```python
from build123d import *

# Parameters (mm, degrees)
SKETCH1_W           = 30
SKETCH1_H           = 15
BOSS_EXTRUDE1_DEPTH = 10
BOSS_EXTRUDE2_DEPTH = 15
FILLET1_R           = 3
SKETCH3_R           = 1.25
CUT_EXTRUDE1_DEPTH  = 11
SKETCH4_R           = 1.25
CUT_EXTRUDE2_DEPTH  = 16.0000001


with BuildPart() as part:
    # Sketch1 → Boss-Extrude1 (new body)
    with BuildSketch(Plane(origin=(0, 0, 0), x_dir=(1, 0, 0), z_dir=(0, 1, 0))):
        Rectangle(SKETCH1_W, SKETCH1_H)
    extrude(amount=BOSS_EXTRUDE1_DEPTH)

    # Sketch2 → Boss-Extrude2 (add)
    with BuildSketch(Plane.XZ):
        Polygon((-13, -5.5), (-4, -5.5), (-4, -1.5), (4, -1.5), (4, -5.5), (13, -5.5), (13, 5.5), (4, 5.5), (4, 1.5), (-4, 1.5), (-4, 5.5), (-13, 5.5), align=None)
    extrude(amount=BOSS_EXTRUDE2_DEPTH)

    # Fillet1
    fillet1_edges = [part.edges().sort_by_distance(p)[0] for p in [
        (-15, 10, 0),
        (0, 10, 7.5),
        (13, -7.5, 5.5),
        (-13, -7.5, 5.5),
        (-13, -7.5, -5.5),
        (13, -7.5, -5.5),
        (15, 10, 0),
        (15, 5, 7.5),
        (-15, 5, 7.5),
        (-15, 5, -7.5),
        (15, 5, -7.5),
        (0, 10, -7.5),
    ]]
    fillet(fillet1_edges, radius=FILLET1_R)

    # Sketch3 → Cut-Extrude1 (cut, through all)
    with BuildSketch(Plane.XZ):
        with Locations((0, 3.5)):
            Circle(SKETCH3_R)
        with Locations((0, -3.5)):
            Circle(SKETCH3_R)
    extrude(amount=-CUT_EXTRUDE1_DEPTH, mode=Mode.SUBTRACT)

    # Sketch4 → Cut-Extrude2 (cut, through all)
    with BuildSketch(Plane.XY.offset(7.5)):
        with Locations((0, 5)):
            Circle(SKETCH4_R)
    extrude(amount=-CUT_EXTRUDE2_DEPTH, mode=Mode.SUBTRACT)


solid = part.part
```
The model under review builds one solid part; all positions refer to its coordinate system, in mm. A direction names the side the tool comes from. Round coordinates to 2 decimals unless told otherwise and drop trailing zeros. Loops run counter-clockwise (first coordinate to the right, second up) from the corner with the lowest first, then second, coordinate; pieces in that order, holes last. Notation, with made-up numbers: (59, 12) - (112, 12) arc R24 ccw to (112, 27) - close; hole circle Ø2 at (68.5, -16.5). An arc over 180 degrees is marked (long way). Write each question's results on one line, items separated by ' | '. Start each with the question number.
Q1. Insertion check: P1, Ø4, axis at x = 1.5, y = -4.5, coming from the -Z side; P2, Ø4, axis at x = -11, y = -5.5, coming from the +Z side; P3, Ø4.5, axis at y = -7.5, z = 2.5, coming from the +X side. Each pin has a flat end and moves straight along its axis. Give the tip position at first contact, or say it passes through.
Q2. Take a section at D-D on y = 1.25. Give the boundary of the cut face in (x, z), plus the area to 3 significant figures.
Q3. Draft analysis for pull direction X (two halves, no side actions). For faces 1 (the cylindrical face through (-1.25, 1.91, -3.45)), 2 (the cylindrical face through (1.155, 4.521, 5.972)), 3 (the cylindrical face through (0.17, 9.1, -6.64)), 4 (the flat face through (-15, 3, 0)), state which applies: pulls with the +X half, pulls with the -X half, needs draft (parallel to the pull), parting line crosses it, or undercut.
Q4. Wall thickness on line 1 along Z through (x, y) = (0, 6.8); line 2 along X through (y, z) = (1.05, 3.5); line 3 along X through (y, z) = (-7.25, 2): over which ranges is each line inside the solid? List them lowest first. Write a range as [from, to].
Q5. Take a section at B-B on y = -5.75. Give the boundary of the cut face in (x, z).
Q6. Take a section at C-C on x = 6.5. Give the boundary of the cut face in (y, z), plus the area to 3 significant figures.
Q7. Tool access review of faces 5 (the flat face through (7, -7, -5.5)), 6 (the flat face through (-7, -7, 5.5)), 7 (the flat face through (4, -7, 4)), 8 (the cylindrical face through (12.14, -7.6, -4.6)): name each direction out of +Z, -Z, +X, -X, +Y, -Y from which nothing blocks a thin tool from reaching the whole face with its end or side.
Q8. Take a section at A-A on z = -0.5. Give the boundary of the cut face in (x, y), plus the area to 3 significant figures.
Data:
1) P1: stops at z = -1.5 | P2: stops at z = 5.5 | P3: stops at x = 13
2) outline: (-15, -4.5) arc R3 ccw to (-12, -7.5) - (12, -7.5) arc R3 ccw to (15, -4.5) - (15, 4.5) arc R3 ccw to (12, 7.5) - (-12, 7.5) arc R3 ccw to (-15, 4.5) - close; hole circle Ø2.5 at (0, -3.5); hole circle Ø2.5 at (0, 3.5) | area: 432 mm²
3) face 1: undercut | face 2: undercut | face 3: needs draft | face 4: pulls with the -X half
4) line 1: z = [-7.5, -4.75], [-2.25, 2.25], [4.75, 7.5] | line 2: x = [-15, -1.25], [1.25, 15] | line 3: x = [-13, -4], [4, 13]
5) outline: (-13, -2.5) arc R3 ccw to (-10, -5.5) - (-4, -5.5) - (-4, -1.5) - (4, -1.5) - (4, -5.5) - (10, -5.5) arc R3 ccw to (13, -2.5) - (13, 2.5) arc R3 ccw to (10, 5.5) - (4, 5.5) - (4, 1.5) - (-4, 1.5) - (-4, 5.5) - (-10, 5.5) arc R3 ccw to (-13, 2.5) - close
6) outline: (-15, -5.5) - (0, -5.5) - (0, -7.5) - (7, -7.5) arc R3 ccw to (10, -4.5) - (10, 4.5) arc R3 ccw to (7, 7.5) - (0, 7.5) - (0, 5.5) - (-15, 5.5) - close | area: 311 mm²
7) face 5: -Z, +X, -X, -Y | face 6: +Z, +X, -X, -Y | face 7: +Z, -Y | face 8: -Z, +X, -Y
8) outline: (-15, 0) - (-13, 0) - (-13, -15) - (13, -15) - (13, 0) - (15, 0) - (15, 7) arc R3 ccw to (12, 10) - (-12, 10) arc R3 ccw to (-15, 7) - close; hole circle Ø2.5 at (0, 5) | area: 681 mm²
